```python
from build123d import *

# Parameters (mm, degrees)
ESQUISSE1_W             = 65
ESQUISSE1_H             = 80
BOSS_EXTRU_1_DEPTH      = 4
ESQUISSE2_R             = 2.1
ENL_V_MAT_EXTRU_1_DEPTH = 52.693810074
ESQUISSE3_R             = 2.1
ESQUISSE3_R_2           = 4
ENL_V_MAT_EXTRU_2_DEPTH = 52.693810074
ESQUISSE4_W             = 1
ESQUISSE4_H             = 80
BOSS_EXTRU_2_DEPTH      = 4


with BuildPart() as part:
    # Esquisse1 → Boss.-Extru.1 (new body)
    with BuildSketch(Plane.XY):
        Rectangle(ESQUISSE1_W, ESQUISSE1_H)
    extrude(amount=BOSS_EXTRU_1_DEPTH)

    # Esquisse2 → Enlèv. mat.-Extru.1 (cut, through all)
    with BuildSketch(Plane(origin=(0, 0, 0), x_dir=(-1, 0, 0), z_dir=(0, 0, -1))):
        with Locations((25.85, -31.43902252)):
            Circle(ESQUISSE2_R)
        with Locations(Location((-25.85, -31.43902252, 0), (0, 0, 180))):
            Circle(ESQUISSE2_R)
    extrude(amount=-ENL_V_MAT_EXTRU_1_DEPTH, mode=Mode.SUBTRACT)

    # Esquisse3 → Enlèv. mat.-Extru.2 (cut, through all)
    with BuildSketch(Plane.XY.offset(4)):
        with Locations((-23.653359533, -20.639976695)):
            Circle(ESQUISSE3_R)
        with Locations((23.426593857, -20.639976695)):
            Circle(ESQUISSE3_R)
        with Locations((23.426593857, 26.439976695)):
            Circle(ESQUISSE3_R)
        with Locations((-23.653359533, 26.439976695)):
            Circle(ESQUISSE3_R)
        with Locations((-0.113382838, 2.9)):
            Circle(ESQUISSE3_R_2)
    extrude(amount=-ENL_V_MAT_EXTRU_2_DEPTH, mode=Mode.SUBTRACT)

    # Esquisse4 → Boss.-Extru.2 (add)
    with BuildSketch(Plane(origin=(0, 0, 0), x_dir=(-1, 0, 0), z_dir=(0, 0, -1))):
        with Locations((33, 0)):
            Rectangle(ESQUISSE4_W, ESQUISSE4_H)
        with Locations((-33, 0)):
            Rectangle(ESQUISSE4_W, ESQUISSE4_H)
    extrude(amount=-BOSS_EXTRU_2_DEPTH)


solid = part.part
```
Work out the finished part from the listing and answer in its coordinate system (mm). Give positions to 0.01 mm unless a question says otherwise; leave off trailing zeros. Order: outer loops, then holes, each group sorted by start corner. A loop starts at its lowest first (then second) coordinate and runs counter-clockwise, first axis right, second up.
1. Section B-B, the plane z = 2.8 is taken. Determine the outline of the cut face in (x, y).
Result sheet:
outline: (-33.5, -40) - (33.5, -40) - (33.5, 40) - (-33.5, 40) - close; hole circle Ø4.2 at (-25.85, -31.44); hole circle Ø4.2 at (-23.65, -20.64); hole circle Ø4.2 at (-23.65, 26.44); hole circle Ø8 at (-0.11, 2.9); hole circle Ø4.2 at (23.43, -20.64); hole circle Ø4.2 at (23.43, 26.44); hole circle Ø4.2 at (25.85, -31.44)
2. The mould has two halves that part along Y. Classify faces 1 (the flat face through (8, 1, 4)), 2 (the cylindrical face through (26.819, -29.576, 1.972)), 3 (the flat face through (0, 40, 2)): released by +Y, released by -Y, zero draft, split by the parting line, or undercut.
Result sheet:
face 1: zero draft
face 2: undercut
face 3: released by +Y
3. Section A-A, the plane y = 2.9 is taken. Determine the outline of the cut face in (x, z).
Result sheet:
outline: (-33.5, 0) - (-4.11, 0) - (-4.11, 4) - (-33.5, 4) - close; (3.89, 0) - (33.5, 0) - (33.5, 4) - (3.89, 4) - close
4. Straight lines are drawn through the part: L1, parallel to Y at x = 21.5, z = 0.9; L2, parallel to Y at x = 23, z = 0.25; L3, parallel to Y at x = -25.85, z = 1.65. For each, find the intervals that lie inside material, in ascending order.
Result sheet:
L1: y = -40 to -21.48, -19.8 to 25.6, 27.28 to 40
L2: y = -40 to -22.7, -18.58 to 24.38, 28.5 to 40
L3: y = -40 to -33.54, -29.34 to 40
